```python
from build123d import *

# Parameters (mm, degrees)
SKETCH2_W                    = 22
SKETCH2_H                    = 10
BOSS_EXTRUDE1_DEPTH          = 0.8128
EDGE_FLANGE1_DEPTH           = 10
EDGE_FLANGE2_DEPTH           = 10
EDGE_FLANGE3_STRIP_W         = 4.8768
EDGE_FLANGE3_STRIP_H         = 0.8128
EDGE_FLANGE3_STRIP_CUT_DEPTH = 10
EDGE_FLANGE3_DEPTH           = 10
EDGE_FLANGE4_STRIP_W         = 4.8768
EDGE_FLANGE4_STRIP_H         = 0.8128
EDGE_FLANGE4_STRIP_CUT_DEPTH = 10
EDGE_FLANGE4_DEPTH           = 10
CUT_EXTRUDE1_REACH           = 40.457
SKETCH21_R                   = 1.5
CUT_EXTRUDE2_REACH           = 40.457
SKETCH22_R                   = 2.25


# Sheet-metal steps are written as plain solids
with BuildPart() as part:
    # Sketch2 → Boss-Extrude1 (new body)
    with BuildSketch(Plane(origin=(0, 0, 0), x_dir=(1, 0, 0), z_dir=(0, 1, 0))):
        with Locations((11, 5)):
            Rectangle(SKETCH2_W, SKETCH2_H)
    extrude(amount=BOSS_EXTRUDE1_DEPTH)

    # Edge-Flange1 section (across the edge) → Edge-Flange1 (add)
    with BuildSketch(Plane(origin=(-0.8128, 0.8128, -10), x_dir=(1, 0, 0), z_dir=(0, 0, 1))):
        with BuildLine():
            Line((-0.8128, 0.8128), (-0.8128, 14.13))
            Line((-0.8128, 14.13), (0, 14.13))
            Line((0, 14.13), (0, 0.8128))
            ThreePointArc((0, 0.8128), (0.238063608, 0.238063608), (0.8128, 0))
            Line((0.8128, 0), (0.8128, -0.8128))
            ThreePointArc((0.8128, -0.8128), (-0.336672783, -0.336672783), (-0.8128, 0.8128))
        make_face()
    extrude(amount=EDGE_FLANGE1_DEPTH)

    # Edge-Flange2 section (across the edge) → Edge-Flange2 (add)
    with BuildSketch(Plane(origin=(22.8128, 0.8128, 0), x_dir=(-1, 0, 0), z_dir=(0, 0, -1))):
        with BuildLine():
            Line((-0.8128, 0.8128), (-0.8128, 14.13))
            Line((-0.8128, 14.13), (0, 14.13))
            Line((0, 14.13), (0, 0.8128))
            ThreePointArc((0, 0.8128), (0.238063608, 0.238063608), (0.8128, 0))
            Line((0.8128, 0), (0.8128, -0.8128))
            ThreePointArc((0.8128, -0.8128), (-0.336672783, -0.336672783), (-0.8128, 0.8128))
        make_face()
    extrude(amount=EDGE_FLANGE2_DEPTH)

    # Edge-Flange3 strip (across the edge) → Edge-Flange3 strip cut (cut)
    with BuildSketch(Plane(origin=(-1.6256, 14.9428, 0), x_dir=(0, -1, 0), z_dir=(0, 0, -1))):
        with Locations((-1.6256, -0.4064)):
            Rectangle(EDGE_FLANGE3_STRIP_W, EDGE_FLANGE3_STRIP_H)
    extrude(amount=EDGE_FLANGE3_STRIP_CUT_DEPTH, mode=Mode.SUBTRACT)

    # Edge-Flange3 section (across the edge) → Edge-Flange3 (add)
    with BuildSketch(Plane(origin=(-1.6256, 14.9428, 0), x_dir=(0, -1, 0), z_dir=(0, 0, -1))):
        with BuildLine():
            Line((-0.8128, 0.8128), (-0.8128, 10.4384))
            Line((-0.8128, 10.4384), (0, 10.4384))
            Line((0, 10.4384), (0, 0.8128))
            ThreePointArc((0, 0.8128), (0.238063608, 0.238063608), (0.8128, 0))
            Line((0.8128, 0), (0.8128, -0.8128))
            ThreePointArc((0.8128, -0.8128), (-0.336672783, -0.336672783), (-0.8128, 0.8128))
        make_face()
    extrude(amount=EDGE_FLANGE3_DEPTH)

    # Edge-Flange4 strip (across the edge) → Edge-Flange4 strip cut (cut)
    with BuildSketch(Plane(origin=(23.6256, 14.9428, -10), x_dir=(0, -1, 0), z_dir=(0, 0, 1))):
        with Locations((-1.6256, -0.4064)):
            Rectangle(EDGE_FLANGE4_STRIP_W, EDGE_FLANGE4_STRIP_H)
    extrude(amount=EDGE_FLANGE4_STRIP_CUT_DEPTH, mode=Mode.SUBTRACT)

    # Edge-Flange4 section (across the edge) → Edge-Flange4 (add)
    with BuildSketch(Plane(origin=(23.6256, 14.9428, -10), x_dir=(0, -1, 0), z_dir=(0, 0, 1))):
        with BuildLine():
            Line((-0.8128, 0.8128), (-0.8128, 10))
            Line((-0.8128, 10), (0, 10))
            Line((0, 10), (0, 0.8128))
            ThreePointArc((0, 0.8128), (0.238063608, 0.238063608), (0.8128, 0))
            Line((0.8128, 0), (0.8128, -0.8128))
            ThreePointArc((0.8128, -0.8128), (-0.336672783, -0.336672783), (-0.8128, 0.8128))
        make_face()
    extrude(amount=EDGE_FLANGE4_DEPTH)

    # Sketch21 → Cut-Extrude1 (cut, up to next)
    with BuildSketch(Plane(origin=(0, 15.7556, 0), x_dir=(1, 0, 0), z_dir=(0, 1, 0)), mode=Mode.PRIVATE) as cut_extrude1_sk1:
        with Locations(Location((-7.2512, 5, 0), (0, 0, 270))):
            Circle(SKETCH21_R)
    cut_extrude1_tool1 = extrude(cut_extrude1_sk1.sketch, amount=-CUT_EXTRUDE1_REACH, mode=Mode.PRIVATE) & part.part
    # Sketch21 → Cut-Extrude1 (cut, up to next)
    with BuildSketch(Plane(origin=(0, 15.7556, 0), x_dir=(1, 0, 0), z_dir=(0, 1, 0)), mode=Mode.PRIVATE) as cut_extrude1_sk2:
        with Locations(Location((29.2512, 5, 0), (0, 0, 90))):
            Circle(SKETCH21_R)
    cut_extrude1_tool2 = extrude(cut_extrude1_sk2.sketch, amount=-CUT_EXTRUDE1_REACH, mode=Mode.PRIVATE) & part.part
    add(cut_extrude1_tool1.solids().sort_by_distance((-7.2512, 15.7556, -5))[0], mode=Mode.SUBTRACT)
    add(cut_extrude1_tool2.solids().sort_by_distance((29.2512, 15.7556, -5))[0], mode=Mode.SUBTRACT)

    # Sketch22 → Cut-Extrude2 (cut, up to next)
    with BuildSketch(Plane.XZ, mode=Mode.PRIVATE) as cut_extrude2_sk1:
        with Locations(Location((6, -5, 0), (0, 0, 270))):
            Circle(SKETCH22_R)
    cut_extrude2_tool1 = extrude(cut_extrude2_sk1.sketch, amount=-CUT_EXTRUDE2_REACH, mode=Mode.PRIVATE) & part.part
    # Sketch22 → Cut-Extrude2 (cut, up to next)
    with BuildSketch(Plane.XZ, mode=Mode.PRIVATE) as cut_extrude2_sk2:
        with Locations(Location((16, -5, 0), (0, 0, 270))):
            Circle(SKETCH22_R)
    cut_extrude2_tool2 = extrude(cut_extrude2_sk2.sketch, amount=-CUT_EXTRUDE2_REACH, mode=Mode.PRIVATE) & part.part
    add(cut_extrude2_tool1.solids().sort_by_distance((6, 0, -5))[0], mode=Mode.SUBTRACT)
    add(cut_extrude2_tool2.solids().sort_by_distance((16, 0, -5))[0], mode=Mode.SUBTRACT)


solid = part.part
```
Input: part model. Units: mm. Frame: model coordinates. A direction names the side the tool comes from. Round coordinates to 2 decimals unless told otherwise and drop trailing zeros. Order: outer loops, then holes, each group sorted by start corner. A loop starts at its lowest first (then second) coordinate and runs counter-clockwise, first axis right, second up. Notation, with made-up numbers: (40.25, 5) - (84.25, 5) arc R31 cw to (84.25, 41) - close; hole circle Ø8 at (30, -32.5). An arc over 180 degrees is marked (long way). One line per question, with ' | ' between items. Start each with the question number.
1) Pull-direction query (Z, two-part tool) for faces 4 (the flat face through (-1, 7, 0)), 5 (the cylindrical face through (23.137, 0.464, -4.93)), 6 (the cylindrical face through (30.716, 15.355, -4.675)); classes: +Z half, -Z half, draft (parallel to the pull), parting line (faces both ways), or undercut.
2) Contact query for flat-ended pins moving along their axis: P1, Ø1, axis at x = 14, z = -2.5, coming from the -Y side; P2, Ø4, axis at x = 29.25, z = -5, coming from the -Y side; P3, Ø6, axis at y = 6, z = -1.5, coming from the +X side; P4, Ø5, axis at y = 6.5, z = -7, coming from the -X side. Output: stop coordinate, or through.
3) Cut plane A-A, the plane y = 5.25. Return the cut outline in (x, z), then the cut area to 3 significant figures.
4) Cut plane C-C, the plane z = -9. Return the cut outline in (x, y).
5) Cut plane D-D, the plane z = -5. Give the number of separate pieces and of enclosed holes in the cut face, then the cut area to 3 significant figures.
6) Ray query, probe 1 along X at (y, z) = (10, -4.25); probe 2 along Y at (x, z) = (5, -2.25); probe 3 along X at (y, z) = (15.2, -5). Return the intervals inside material, ascending.
7) Cut plane B-B, the plane x = 16. Return the cut outline in (y, z).
8) Set-up query: faces 1 (the flat face through (23.626, 8, -5)), 2 (the flat face through (-1, 7, -10)), 3 (the flat face through (22.813, 8, -5)). Return all of +Z, -Z, +X, -X, +Y, -Y with unobstructed straight access to the full face (end or side cutting, diameter ignored); none if empty.
Worked out:
1) face 4: +Z half | face 5: draft | face 6: undercut
2) P1: stops at y = 0 | P2: stops at y = 14.94 | P3: stops at x = 23.63 | P4: stops at x = -1.63
3) outline: (-1.63, -10) - (-0.81, -10) - (-0.81, 0) - (-1.63, 0) - close; (22.81, -10) - (23.63, -10) - (23.63, 0) - (22.81, 0) - close | area: 16.3 mm^2
4) outline: (-12.06, 14.94) - (-2.44, 14.94) arc R0.81 cw to (-1.63, 14.13) - (-1.63, 1.63) arc R1.63 ccw to (0, 0) - (22, 0) arc R1.63 ccw to (23.63, 1.63) - (23.63, 14.13) arc R0.81 cw to (24.44, 14.94) - (33.63, 14.94) - (33.63, 15.76) - (24.44, 15.76) arc R1.63 ccw to (22.81, 14.13) - (22.81, 1.63) arc R0.81 cw to (22, 0.81) - (0, 0.81) arc R0.81 cw to (-0.81, 1.63) - (-0.81, 14.13) arc R1.63 ccw to (-2.44, 15.76) - (-12.06, 15.76) - close
5) separate pieces: 5 | enclosed holes: 0 | area: 47.5 mm^2
6) probe 1: x = -1.63 to -0.81, 22.81 to 23.63 | probe 2: y = 0 to 0.81 | probe 3: x = -12.06 to -8.75, -5.75 to -1.21, 23.21 to 27.75, 30.75 to 33.63
7) outline: (0, -10) - (0.81, -10) - (0.81, -7.25) - (0, -7.25) - close; (0, -2.75) - (0.81, -2.75) - (0.81, 0) - (0, 0) - close
8) face 1: +Z, -Z, +X, -Y | face 2: -Z, +X, -X, +Y, -Y | face 3: +Z, -Z, +Y
